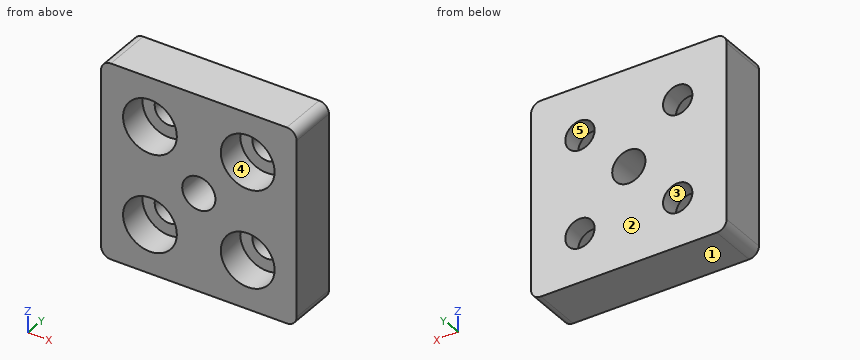
```python
from build123d import *

# Parameters (mm, degrees)
SKETCH_1_R             = 3
EXTRUDE_1_DEPTH        = 10
SKETCH_3_R             = 5.5
CUT_EXTRUDE_1_DEPTH    = 6
HOLE_WIZARD_M8_1_D     = 6.8
HOLE_WIZARD_M8_1_DEPTH = 38.75
HOLE_WIZARD_M8_1_TIP   = 2.042926105


with BuildPart() as part:
    # 草图1 → 凸台-拉伸1 (new body)
    with BuildSketch(Plane(origin=(0, 0, 0), x_dir=(1, 0, 0), z_dir=(0, 1, 0))):
        with BuildLine():
            Line((-18, 0), (18, 0))
            ThreePointArc((18, 0), (19.414213562, 0.585786438), (20, 2))
            Line((20, 2), (20, 38))
            ThreePointArc((20, 38), (19.414213562, 39.414213562), (18, 40))
            Line((18, 40), (-18, 40))
            ThreePointArc((-18, 40), (-19.414213562, 39.414213562), (-20, 38))
            Line((-20, 38), (-20, 2))
            ThreePointArc((-20, 2), (-19.414213562, 0.585786438), (-18, 0))
        make_face()
        with Locations(Location((10, 30, 0), (0, 0, 270))):
            Circle(SKETCH_1_R, mode=Mode.SUBTRACT)
        with Locations(Location((-10, 30, 0), (0, 0, 270))):
            Circle(SKETCH_1_R, mode=Mode.SUBTRACT)
        with Locations(Location((-10, 10, 0), (0, 0, 270))):
            Circle(SKETCH_1_R, mode=Mode.SUBTRACT)
        with Locations(Location((10, 10, 0), (0, 0, 270))):
            Circle(SKETCH_1_R, mode=Mode.SUBTRACT)
    extrude(amount=EXTRUDE_1_DEPTH)

    # 草图3 → 切除-拉伸1 (cut)
    with BuildSketch(Plane.XZ):
        with Locations(Location((-10, -10, 0), (0, 0, 270))):
            Circle(SKETCH_3_R)
        with Locations(Location((10, -10, 0), (0, 0, 270))):
            Circle(SKETCH_3_R)
        with Locations(Location((10, -30, 0), (0, 0, 270))):
            Circle(SKETCH_3_R)
        with Locations(Location((-10, -30, 0), (0, 0, 270))):
            Circle(SKETCH_3_R)
    extrude(amount=-CUT_EXTRUDE_1_DEPTH, mode=Mode.SUBTRACT)

    # M8 螺纹孔1
    with Locations(Plane(origin=(0, 10, -20), x_dir=(0, 0, 1), z_dir=(0, 1, 0))):
        with Locations((0, 0)):
            Hole(HOLE_WIZARD_M8_1_D / 2, depth=HOLE_WIZARD_M8_1_DEPTH)
            with Locations((0, 0, -(HOLE_WIZARD_M8_1_DEPTH + HOLE_WIZARD_M8_1_TIP / 2))):  # 118° drill point
                Cone(0, HOLE_WIZARD_M8_1_D / 2, HOLE_WIZARD_M8_1_TIP, mode=Mode.SUBTRACT)


solid = part.part
```
Here's how the part is built. I have some questions about the finished solid (model axes, mm). Face numbers are marked on the shaded views. A direction names the side the tool comes from. Round coordinates to 2 decimals unless told otherwise and drop trailing zeros. Loops run counter-clockwise (first coordinate to the right, second up) from the corner with the lowest first, then second, coordinate; pieces in that order, holes last.
1. Thinking about a two-plate mould opening in Z: for the marked faces 1, 2 and 3, which applies, released by +Z, released by -Z, zero draft, split by the parting line, or undercut?
Answers:
face 1: released by -Z
face 2: zero draft
face 3: undercut
2. Suppose I cut it at D-D, the plane z = -10. Please give me the cut outline in (x, y), and give its area (3 significant figures).
Answers:
outline: (-20, 0) - (-15.5, 0) - (-15.5, 6) - (-13, 6) - (-13, 10) - (-20, 10) - close; (-7, 6) - (-4.5, 6) - (-4.5, 0) - (4.5, 0) - (4.5, 6) - (7, 6) - (7, 10) - (-7, 10) - close; (13, 6) - (15.5, 6) - (15.5, 0) - (20, 0) - (20, 10) - (13, 10) - close
area: 220 mm2
3. Suppose I cut it at B-B, the plane y = 8.5. Please give me the cut outline in (x, z).
Answers:
outline: (-20, -38) arc R2 ccw to (-18, -40) - (18, -40) arc R2 ccw to (20, -38) - (20, -2) arc R2 ccw to (18, 0) - (-18, 0) arc R2 ccw to (-20, -2) - close; hole circle Ø6 at (-10, -30); hole circle Ø6 at (-10, -10); hole circle Ø6.8 at (0, -20); hole circle Ø6 at (10, -30); hole circle Ø6 at (10, -10)
4. For the marked faces 4 and 5, which set-ups out of +Z, -Z, +X, -X, +Y, -Y let a thin tool reach every point of the face, with its end or its side?
Answers:
face 4: -Y
face 5: +Y, -Y
5. Suppose I cut it at C-C, the plane x = 10. Please give me the cut outline in (y, z), and give its area (3 significant figures).
Answers:
outline: (0, -40) - (10, -40) - (10, -33) - (6, -33) - (6, -35.5) - (0, -35.5) - close; (0, -24.5) - (6, -24.5) - (6, -27) - (10, -27) - (10, -13) - (6, -13) - (6, -15.5) - (0, -15.5) - close; (0, -4.5) - (6, -4.5) - (6, -7) - (10, -7) - (10, 0) - (0, 0) - close
area: 220 mm2
6. Will these pins go through, and if not, where does the flat tip stop? pin 1 (10 mm diameter, centred on x = 10.5, z = -8.5, fed in from +Y); pin 2 (5.5 mm diameter, centred on x = 9, z = -31, fed in from -Y).
Answers:
pin 1: stops at y = 10
pin 2: stops at y = 6
7. If I drill on probe 1 along X at (y, z) = (4.15, -10); probe 2 along X at (y, z) = (9.05, -10); probe 3 along Z at (x, y) = (-10, 9.1), over which ranges is the centre line in solid material (lowest first)?
Answers:
probe 1: x = -20 to -15.5, -4.5 to 4.5, 15.5 to 20
probe 2: x = -20 to -13, -7 to 7, 13 to 20
probe 3: z = -40 to -33, -27 to -13, -7 to 0
8. Suppose I cut it at A-A, the plane z = -20. Please give me the cut outline in (x, y), and give its area (3 significant figures).
Answers:
outline: (-20, 0) - (-3.4, 0) - (-3.4, 10) - (-20, 10) - close; (3.4, 0) - (20, 0) - (20, 10) - (3.4, 10) - close
area: 332 mm2
